```python
from build123d import *

# Parameters (mm, degrees)
SKETCH1_W            = 40.5
SKETCH1_H            = 20
BOSS_EXTRUDE1_DEPTH  = 37.5
BOSS_EXTRUDE2_DEPTH  = 2
SKETCH3_R            = 6.4
BOSS_EXTRUDE3_DEPTH  = 1
SKETCH4_R            = 5.575
BOSS_EXTRUDE4_DEPTH  = 0.5
BOSS_EXTRUDE5_DEPTH  = 2.5
MIRROR2_COPY_1_DEPTH = 2.5
SKETCH_1_W           = 7
SKETCH_1_H           = 2.5
CUT_EXTRUDE_1_DEPTH  = 53.768953941


with BuildPart() as part:
    # Sketch1 → Boss-Extrude1 (new body)
    with BuildSketch(Plane(origin=(0, 0, 0), x_dir=(1, 0, 0), z_dir=(0, 1, 0))):
        Rectangle(SKETCH1_W, SKETCH1_H)
    extrude(amount=BOSS_EXTRUDE1_DEPTH)

    # Sketch2 → Boss-Extrude2 (add)
    with BuildSketch(Plane(origin=(0, 37.5, 0), x_dir=(1, 0, 0), z_dir=(0, 1, 0))):
        with BuildLine():
            Line((-4.95, -9), (14.25, -9))
            Line((14.25, -9), (14.25, -4.8))
            ThreePointArc((14.25, -4.8), (16.65, 0), (14.25, 4.8))
            Line((14.25, 4.8), (14.25, 9))
            Line((14.25, 9), (-4.95, 9))
            ThreePointArc((-4.95, 9), (-19.308898944, 0), (-4.95, -9))
        make_face()
    extrude(amount=BOSS_EXTRUDE2_DEPTH)

    # Sketch3 → Boss-Extrude3 (add)
    with BuildSketch(Plane(origin=(0, 39.5, 0), x_dir=(1, 0, 0), z_dir=(0, 1, 0))):
        with Locations(Location((-9.308898944, 0, 0), (0, 0, 270))):
            Circle(SKETCH3_R)
    extrude(amount=BOSS_EXTRUDE3_DEPTH)

    # Sketch4 → Boss-Extrude4 (add)
    with BuildSketch(Plane(origin=(0, 40.5, 0), x_dir=(1, 0, 0), z_dir=(0, 1, 0))):
        with Locations(Location((-9.308898944, 0, 0), (0, 0, 270))):
            Circle(SKETCH4_R)
    extrude(amount=BOSS_EXTRUDE4_DEPTH)

    # Sketch5 → Boss-Extrude5 (add)
    with BuildSketch(Plane(origin=(0, 31.2, 0), x_dir=(1, 0, 0), z_dir=(0, 1, 0))):
        with BuildLine():
            Line((20.25, 9), (27.25, 9))
            Line((27.25, 9), (27.25, 6.25))
            Line((27.25, 6.25), (26.177050983, 6.25))
            ThreePointArc((26.177050983, 6.25), (22.25, 4.75), (26.177050983, 3.25))
            Line((26.177050983, 3.25), (27.25, 3.25))
            Line((27.25, 3.25), (27.25, 0))
            Line((27.25, 0), (20.25, 0))
            Line((20.25, 0), (20.25, 9))
        make_face()
    boss_extrude5 = extrude(amount=-BOSS_EXTRUDE5_DEPTH)

    # Mirror1: Boss-Extrude5 across plane
    add(boss_extrude5.mirror(Plane(origin=(0, 0, 0), x_dir=(0, 0, 1), z_dir=(1, 0, 0))))

    # Mirror2: Boss-Extrude5 across plane
    add(boss_extrude5.mirror(Plane.XY))

    # Mirror2 copy 1 sketch → Mirror2 copy 1 (add)
    with BuildSketch(Plane(origin=(0, 31.2, 0), x_dir=(-1, 0, 0), z_dir=(0, 1, 0))):
        with BuildLine():
            Line((20.25, 9), (27.25, 9))
            Line((27.25, 9), (27.25, 6.25))
            Line((27.25, 6.25), (26.177050983, 6.25))
            ThreePointArc((26.177050983, 6.25), (22.25, 4.75), (26.177050983, 3.25))
            Line((26.177050983, 3.25), (27.25, 3.25))
            Line((27.25, 3.25), (27.25, 0))
            Line((27.25, 0), (20.25, 0))
            Line((20.25, 0), (20.25, 9))
        make_face()
    extrude(amount=-MIRROR2_COPY_1_DEPTH)

    # ｽｹｯﾁ1 → ｶｯﾄ - 押し出し1 (cut, through all)
    with BuildSketch(Plane.XY.offset(9)):
        with Locations((-23.75, 29.95)):
            Rectangle(SKETCH_1_W, SKETCH_1_H)
    extrude(amount=-CUT_EXTRUDE_1_DEPTH, mode=Mode.SUBTRACT)


solid = part.part
```
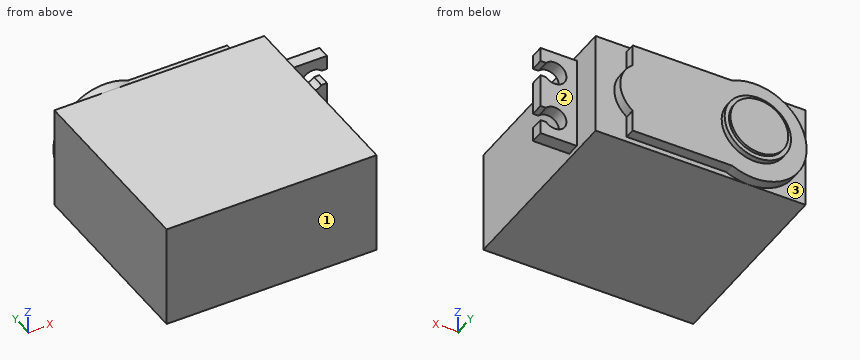
Verification items for the finished model (mm, model axes). Face numbers are marked on the shaded views. A direction names the side the tool comes from. Round coordinates to 2 decimals unless told otherwise and drop trailing zeros. Order: outer loops, then holes, each group sorted by start corner. A loop starts at its lowest first (then second) coordinate and runs counter-clockwise, first axis right, second up.
1) Cross-section at D-D, the plane y = 27. Record the cut outline in (x, z).
Geometry says:
outline: (-20.25, -10) - (20.25, -10) - (20.25, 10) - (-20.25, 10) - close
2) Cross-section at C-C, the plane x = 12.5. Record the cut outline in (y, z).
Geometry says:
outline: (0, -10) - (37.5, -10) - (37.5, -9) - (39.5, -9) - (39.5, 9) - (37.5, 9) - (37.5, 10) - (0, 10) - close
3) Depth check by flat-ended pin: pin 1 (5.5 mm diameter, centred on x = 25, z = 4, fed in from +Y); pin 2 (1 mm diameter, centred on y = 38.5, z = -6, fed in from +X); pin 3 (2 mm diameter, centred on x = 23.5, y = 30, fed in from +Z). Enter the tip coordinate at first touch or a pass-through.
Geometry says:
pin 1: stops at y = 31.2
pin 2: stops at x = 14.25
pin 3: stops at z = 9
4) Material ranges on line 1 (Z direction, x = 24.5, y = 29.4); line 2 (Z direction, x = 24, y = 29); line 3 (X direction, y = 17.5, z = -6.5), recorded low to high.
Geometry says:
line 1: z = -9 to -7, -2.5 to 2.5, 7 to 9
line 2: z = -9 to -6.94, -2.56 to 2.56, 6.94 to 9
line 3: x = -20.25 to 20.25
5) Cross-section at A-A, the plane x = 24.5. Record the cut outline in (y, z).
Geometry says:
outline: (28.7, -9) - (31.2, -9) - (31.2, -7) - (28.7, -7) - close; (28.7, -2.5) - (31.2, -2.5) - (31.2, 2.5) - (28.7, 2.5) - close; (28.7, 7) - (31.2, 7) - (31.2, 9) - (28.7, 9) - close
6) Tool access check on the marked faces 1, 2 and 3. Record the directions out of +Z, -Z, +X, -X, +Y, -Y that give a thin tool (end or side, any length) a straight path to the whole face; none if there is none.
Geometry says:
face 1: +Z, -Z, +X, -X, -Y
face 2: +Z, -Z, +X, +Y
face 3: -X, +Y
7) Cross-section at B-B, the plane z = 0. Record the cut outline in (x, y), plus the area to 3 significant figures.
Geometry says:
outline: (-20.25, 0) - (20.25, 0) - (20.25, 28.7) - (27.25, 28.7) - (27.25, 31.2) - (20.25, 31.2) - (20.25, 37.5) - (16.65, 37.5) - (16.65, 39.5) - (-2.91, 39.5) - (-2.91, 40.5) - (-3.73, 40.5) - (-3.73, 41) - (-14.88, 41) - (-14.88, 40.5) - (-15.71, 40.5) - (-15.71, 39.5) - (-19.31, 39.5) - (-19.31, 37.5) - (-20.25, 37.5) - close
area: 1,630 mm2
